Input: part model. Units: mm. Frame: model coordinates. A direction names the side the tool comes from. Round coordinates to 2 decimals unless told otherwise and drop trailing zeros. Order: outer loops, then holes, each group sorted by start corner. A loop starts at its lowest first (then second) coordinate and runs counter-clockwise, first axis right, second up. Notation, with made-up numbers: M -25,48 L -11,48 A14 cw -11,61 Z; hole C -25.75,-8 d3. An arc over 180 degrees is marked long. One line per question, with ' | ' between items.
Autodesk Inventor part; units mm, degrees
ref_plane "YZ Plane" through (0, 0, 0) normal (1, 0, 0) x (0, 1, 0)
ref_plane "XZ Plane" through (0, 0, 0) normal (0, 1, 0) x (-1, 0, 0)
ref_plane "XY Plane" through (0, 0, 0) normal (0, 0, 1) x (1, 0, 0)
sketch "Эскиз1" plane through (0, 0, 0) normal (0, 1, 0) x (-1, 0, 0)
  line L0 (-250, -250) -> (250, -250)
  line L1 (250, -250) -> (250, 250)
  line L2 (250, 250) -> (-250, 250)
  line L3 (-250, 250) -> (-250, -250)
  line L4 (-250, -250) -> (250, 250) construction
  line L5 (250, -250) -> (-250, 250) construction
  point P0 (0, 0)
  dimension "d0" = 500
  dimension "d1" = 500
extrude "Выдавливание1" add sketch "Эскиз1" along normal blind 20
sketch "Эскиз2" plane through (0, 20, 0) normal (0, 1, 0) x (1, 0, 0)
  line L0 (-250, 250) -> (-250, -250)
  line L1 (250, 250) -> (-250, 250)
  line L2 (-250, 250) -> (-250, -250)
  line L3 (-250, -250) -> (250, -250)
  line L4 (250, -250) -> (250, 250)
  line L5 (250, 250) -> (-250, -250) construction
  line L6 (-250, 250) -> (250, -250) construction
  line L7 (240, 240) -> (-240, 240)
  line L8 (-240, 240) -> (-240, -240)
  line L9 (-240, -240) -> (240, -240)
  line L10 (240, -240) -> (240, 240)
  line L11 (240, 240) -> (-240, -240) construction
  line L12 (-240, 240) -> (240, -240) construction
  point P0 (0, 0)
  dimension "d4" = 480
  dimension "d5" = 480
extrude "Выдавливание2" add sketch "Эскиз2" along normal blind 40
Item 1: First-contact query: pin 1 (1.5 mm diameter, centred on x = 196, z = 31.5, fed in from +Y). Flat tip, straight axial feed; report the tip coordinate or a pass-through.
Report:
pin 1: y = 20
Item 2: Section query B-B, the plane z = -140. Return loops of the section in (x, y), plus the area to 3 significant figures.
Report:
outline: M -250,0 L 250,0 L 250,60 L 240,60 L 240,20 L -240,20 L -240,60 L -250,60 Z | area: 10,800 mm²
Item 3: Mould query, pull axis Z, two halves, no side actions, for faces 1 (the flat face through (3, 30, -250)), 2 (the flat face through (3, 20, 3)), 3 (the flat face through (250, 30, 3)), 4 (the flat face through (-3, 30, 250)). Classes: +Z half, -Z half, draft (parallel to the pull), parting line (faces both ways), or undercut.
Report:
face 1: -Z half | face 2: undercut | face 3: draft | face 4: +Z half
Item 4: Line query: line 1 along X through (y, z) = (37, -78); line 2 along Y through (x, z) = (-151, -49.5). Output: solid intervals per line, ascending. Write a range as from..to.
Report:
line 1: -250..-240, 240..250 | line 2: 0..20
Item 5: Access query for faces 5 (the flat face through (-250, 30, -3)), 6 (the flat face through (-240, 40, -3)). Directions: +Z, -Z, +X, -X, +Y, -Y. A direction counts if a zero-diameter tool reaches every point of the face in a straight line with its end or side. Return the directions, or none.
Report:
face 5: +Z, -Z, -X, +Y, -Y | face 6: +Y
Item 6: Section query C-C, the plane x = -81. Return loops of the section in (y, z).
Report:
outline: M 0,-250 L 60,-250 L 60,-240 L 20,-240 L 20,240 L 60,240 L 60,250 L 0,250 Z
Item 7: Section query A-A, the plane y = 28. Return loops of the section in (x, z), plus the area to 3 significant figures.
Report:
outline: M -250,-250 L 250,-250 L 250,250 L -250,250 Z; hole M -240,-240 L 240,-240 L 240,240 L -240,240 Z | area: 19,600 mm²
